Input: dimensioned drawing with shaded views. Units: mm. Origin: part minimum x, y, z. A direction names the side the tool comes from. Round coordinates to 2 decimals unless told otherwise and drop trailing zeros. Loops run counter-clockwise (first coordinate to the right, second up) from the corner with the lowest first, then second, coordinate; pieces in that order, holes last. Notation, with made-up numbers: M 10,70 L 42,70 A18 cw 42,92 Z; hole C -6,-20.75 d1. An arc over 180 degrees is marked long. One line per item, written item: value.
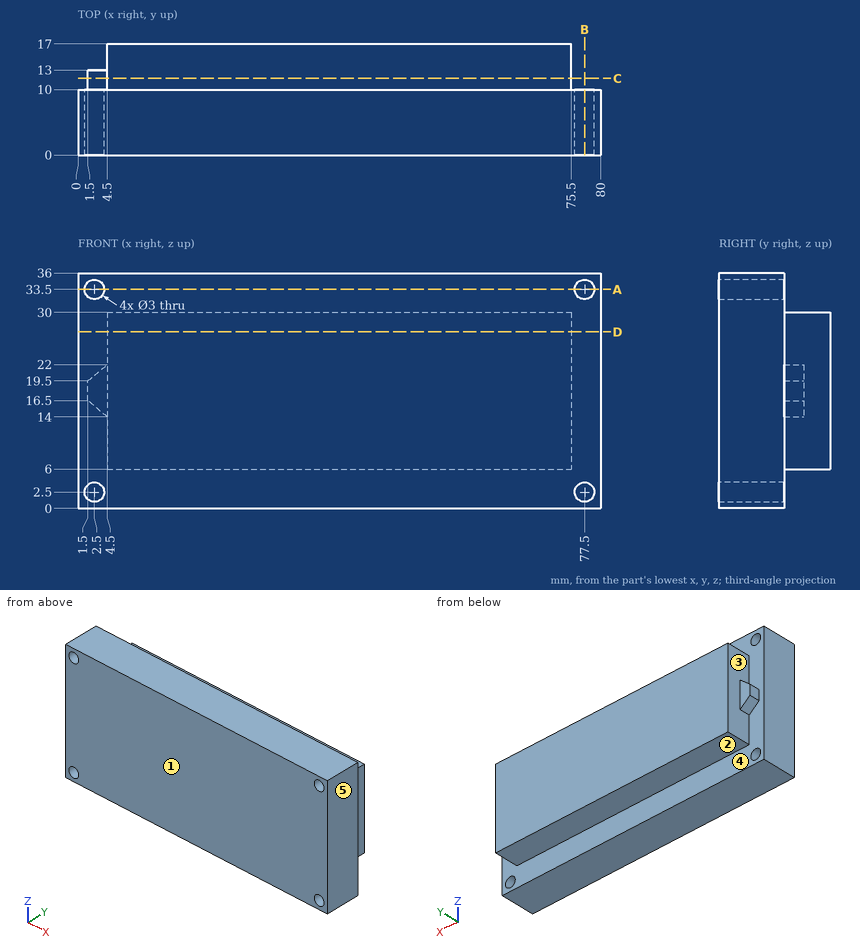
1. Section query B-B (x = 77.5). Return the cut outline in (y, z), and give its area (3 significant figures).
Report:
outline: M 0,0 L 10,0 L 10,1 L 0,1 Z; M 0,4 L 10,4 L 10,32 L 0,32 Z; M 0,35 L 10,35 L 10,36 L 0,36 Z
area: 300 mm2
2. Section query D-D (z = 27). Return the cut outline in (x, y).
Report:
outline: M 0,0 L 80,0 L 80,10 L 75.5,10 L 75.5,17 L 4.5,17 L 4.5,10 L 0,10 Z
3. Ray query, line 1 (X direction, y = 7, z = 2.5); line 2 (Z direction, x = 2.5, y = 3.25); line 3 (X direction, y = 4.75, z = 33). Return the intervals inside material, ascending. Write a range as [from, to].
Report:
line 1: x = [0, 1], [4, 76], [79, 80]
line 2: z = [0, 1], [4, 32], [35, 36]
line 3: x = [0, 1.09], [3.91, 76.09], [78.91, 80]
4. Section query C-C (y = 11.75). Return the cut outline in (x, z), and give its area (3 significant figures).
Report:
outline: M 1.5,16.5 L 4.5,14 L 4.5,6 L 75.5,6 L 75.5,30 L 4.5,30 L 4.5,22 L 1.5,19.5 Z
area: 1,720 mm2
5. Reachability of the marked faces 1 and 2 from +Z, -Z, +X, -X, +Y, -Y: full face, straight path, thin tool, end or side. Return the list, or none.
Report:
face 1: +Z, -Z, +X, -X, -Y
face 2: -Z, +X, -X, +Y
6. Section query A-A (z = 33.5). Return the cut outline in (x, y).
Report:
outline: M 0,0 L 1,0 L 1,10 L 0,10 Z; M 4,0 L 76,0 L 76,10 L 4,10 Z; M 79,0 L 80,0 L 80,10 L 79,10 Z
7. Pull-direction query (X, two-part tool) for the marked faces 3, 4 and 5; classes: released by +X, released by -X, zero draft, split by the parting line, or undercut.
Report:
face 3: released by -X
face 4: zero draft
face 5: released by +X
8. Pin query (flat end, axial travel): pin 1 (4 mm diameter, centred on x = 2.5, z = 33.5, fed in from +Y); pin 2 (5 mm diameter, centred on x = 59, y = 14, fed in from -Z); pin 3 (2.5 mm diameter, centred on x = 77.5, z = 33.5, fed in from -Y); pin 4 (6 mm diameter, centred on x = 47.5, y = 15, fed in from +Z). Return the tip coordinate at first contact, or that it passes through.
Report:
pin 1: stops at y = 10
pin 2: stops at z = 6
pin 3: passes through
pin 4: stops at z = 30
